Verification items for the finished model (mm, model axes). A direction names the side the tool comes from. Give positions to 0.01 mm unless a question says otherwise; leave off trailing zeros. Loops run counter-clockwise (first coordinate to the right, second up) from the corner with the lowest first, then second, coordinate; pieces in that order, holes last. Notation, with made-up numbers: M 30,22 L 54,22 A17 cw 54,52 Z; hole C -35.75,7.5 d2. An arc over 180 degrees is marked long. Answer in a Markdown table with one row per item.
Autodesk Inventor part; units mm, degrees
ref_plane "YZ Plane" through (0, 0, 0) normal (1, 0, 0) x (0, 1, 0)
ref_plane "XZ Plane" through (0, 0, 0) normal (0, 1, 0) x (-1, 0, 0)
ref_plane "XY Plane" through (0, 0, 0) normal (0, 0, 1) x (1, 0, 0)
sketch "スケッチ1" plane through (0, 0, 0) normal (0, 0, 1) x (1, 0, 0)
  circle A0 centre (0, 0) radius 2
  dimension "d0" = 4
extrude "押し出し1" add sketch "スケッチ1" along normal blind 6
sketch "スケッチ2" plane through (0, 0, 6) normal (0, 0, 1) x (1, 0, 0)
  circle A0 centre (0, 0) radius 2
  circle A1 centre (0, 0) radius 4
  dimension "d3" = 8
extrude "押し出し2" add sketch "スケッチ2" along normal blind 3 contours A0 | A1
fillet "フィレット1" radius 3 1 edges at (-4, 0, 9)
thread "ねじ1"
sketch "スケッチ3" plane through (0, 0, 0) normal (0, 0, -1) x (-1, 0, 0)
  circle A0 centre (0, 0) radius 2
extrude "押し出し3" add sketch "スケッチ3" along normal blind 6
properties part number "SB　M4 12mm なべネジ" material "Stainless Steel, 440C"
Item 1: Tool access check on faces 1 (the flat face through (-2, -1, 6)), 2 (the flat face through (0, 0, -6)). Record the directions out of +Z, -Z, +X, -X, +Y, -Y that give a thin tool (end or side, any length) a straight path to the whole face; none if there is none.
Reported:
| item | result |
|---|---|
| face 1 | -Z |
| face 2 | -Z, +X, -X, +Y, -Y |
Item 2: Sectioned sample at A-A (z = 0.25). Record the cut outline in (x, y), and give its area (3 significant figures).
Reported:
| item | result |
|---|---|
| outline | C 0,0 d4 |
| area | 12.6 mm^2 |
Item 3: Go/stop test with a flat-tipped pin: pin 1 (4 mm diameter, centred on x = -0.5, z = -2, fed in from -Y). Record where the tip stops, or that it passes through.
Reported:
| item | result |
|---|---|
| pin 1 | stops at y = -2 |
Item 4: Scan lines: L1, parallel to Y at x = 0, z = -3.25; L2, parallel to Y at x = 0.25, z = 6.75; L3, parallel to Z at x = 2.5, y = -1.75. Record each from-to range of solid material in increasing order. Write a range as [from, to].
Reported:
| item | result |
|---|---|
| L1 | y = [-2, 2] |
| L2 | y = [-3.9, 3.9] |
| L3 | z = [6, 8.19] |
